Part model, mm, in its own coordinate system. Give positions to 0.01 mm unless a question says otherwise; leave off trailing zeros. Order: outer loops, then holes, each group sorted by start corner. A loop starts at its lowest first (then second) coordinate and runs counter-clockwise, first axis right, second up. Notation, with made-up numbers: M 74,36.25 L 128,36.25 A29 cw 128,63.25 Z; hole C 70,70 d4. An arc over 180 degrees is marked long. Answer as a JSON object with one key per item and string values.
from build123d import *

# Parameters (mm, degrees)
SKETCH_1_R      = 2.5
EXTRUDE_1_DEPTH = 22


with BuildPart() as part:
    # 스케치1 → 보스-돌출1 (new body)
    with BuildSketch(Plane.XY):
        Polygon((124.264068712, 300), (-124.264068712, 300), (-300, 124.264068712), (-300, -124.264068712), (-124.264068712, -300), (124.264068712, -300), (300, -124.264068712), (300, 124.264068712), align=None)
        with Locations((0, 290)):
            Circle(SKETCH_1_R, mode=Mode.SUBTRACT)
        with Locations((80, 290)):
            Circle(SKETCH_1_R, mode=Mode.SUBTRACT)
        with Locations((-80, 290)):
            Circle(SKETCH_1_R, mode=Mode.SUBTRACT)
        with Locations((148.492424049, 261.629509039)):
            Circle(SKETCH_1_R, mode=Mode.SUBTRACT)
        with Locations((205.060966544, 205.060966544)):
            Circle(SKETCH_1_R, mode=Mode.SUBTRACT)
        with Locations((261.629509039, 148.492424049)):
            Circle(SKETCH_1_R, mode=Mode.SUBTRACT)
        with Locations((290, 80)):
            Circle(SKETCH_1_R, mode=Mode.SUBTRACT)
        with Locations((290, 0)):
            Circle(SKETCH_1_R, mode=Mode.SUBTRACT)
        with Locations((290, -80)):
            Circle(SKETCH_1_R, mode=Mode.SUBTRACT)
        with Locations((261.629509039, -148.492424049)):
            Circle(SKETCH_1_R, mode=Mode.SUBTRACT)
        with Locations((205.060966544, -205.060966544)):
            Circle(SKETCH_1_R, mode=Mode.SUBTRACT)
        with Locations((148.492424049, -261.629509039)):
            Circle(SKETCH_1_R, mode=Mode.SUBTRACT)
        with Locations((80, -290)):
            Circle(SKETCH_1_R, mode=Mode.SUBTRACT)
        with Locations((0, -290)):
            Circle(SKETCH_1_R, mode=Mode.SUBTRACT)
        with Locations((-80, -290)):
            Circle(SKETCH_1_R, mode=Mode.SUBTRACT)
        with Locations((-148.492424049, -261.629509039)):
            Circle(SKETCH_1_R, mode=Mode.SUBTRACT)
        with Locations((-205.060966544, -205.060966544)):
            Circle(SKETCH_1_R, mode=Mode.SUBTRACT)
        with Locations((-261.629509039, -148.492424049)):
            Circle(SKETCH_1_R, mode=Mode.SUBTRACT)
        with Locations((-290, -80)):
            Circle(SKETCH_1_R, mode=Mode.SUBTRACT)
        with Locations((-290, 0)):
            Circle(SKETCH_1_R, mode=Mode.SUBTRACT)
        with Locations((-290, 80)):
            Circle(SKETCH_1_R, mode=Mode.SUBTRACT)
        with Locations((-261.629509039, 148.492424049)):
            Circle(SKETCH_1_R, mode=Mode.SUBTRACT)
        with Locations((-205.060966544, 205.060966544)):
            Circle(SKETCH_1_R, mode=Mode.SUBTRACT)
        with Locations((-148.492424049, 261.629509039)):
            Circle(SKETCH_1_R, mode=Mode.SUBTRACT)
    extrude(amount=EXTRUDE_1_DEPTH)


solid = part.part
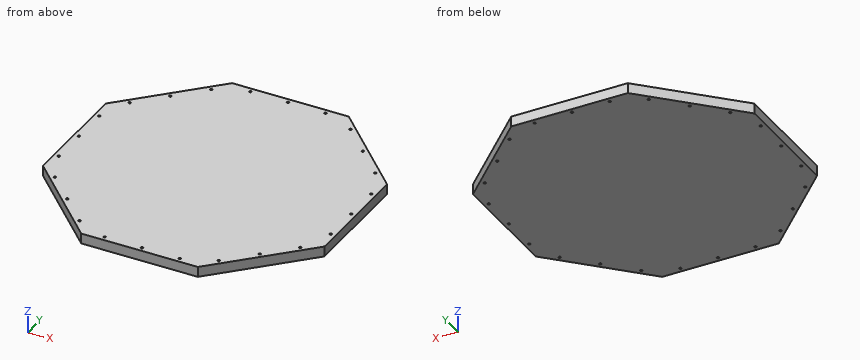
1. Probe line 1 along Y through (x, z) = (79.5, 15.75); line 2 along Y through (x, z) = (-290, 13); line 3 along X through (y, z) = (247.5, 20.5). List the from-to ranges inside material, lowest first.
Worked answers:
{"line 1": "y = -300 to -292.45, -287.55 to 287.55, 292.45 to 300", "line 2": "y = -134.26 to -82.5, -77.5 to -2.5, 2.5 to 77.5, 82.5 to 134.26", "line 3": "x = -176.76 to 176.76"}
2. Pin check, flat tips, straight feed: P1, Ø1.5, axis at x = -232, z = 2.5, coming from the -Y side; P2, Ø2, axis at x = 132.5, z = 18, coming from the +Y side; P3, Ø5, axis at y = -133.5, z = 11, coming from the +X side. Stop position of each tip, or through.
Worked answers:
{"P1": "stops at y = -193.01", "P2": "stops at y = 292.76", "P3": "stops at x = 293.26"}
3. Cut at A-A on z = 16.5. State how many separate pieces and enclosed holes the cut face has, plus the area to 3 significant figures.
Worked answers:
{"separate pieces": "1", "enclosed holes": "24", "area": "298,000 mm^2"}
4. Cut at C-C on y = 226. Give the cut face in (x, z), plus the area to 3 significant figures.
Worked answers:
{"outline": "M -198.26,0 L 198.26,0 L 198.26,22 L -198.26,22 Z", "area": "8,720 mm^2"}
5. Cut at B-B on y = -184.5. Give the cut face in (x, z), plus the area to 3 significant figures.
Worked answers:
{"outline": "M -239.76,0 L 239.76,0 L 239.76,22 L -239.76,22 Z", "area": "10,500 mm^2"}
